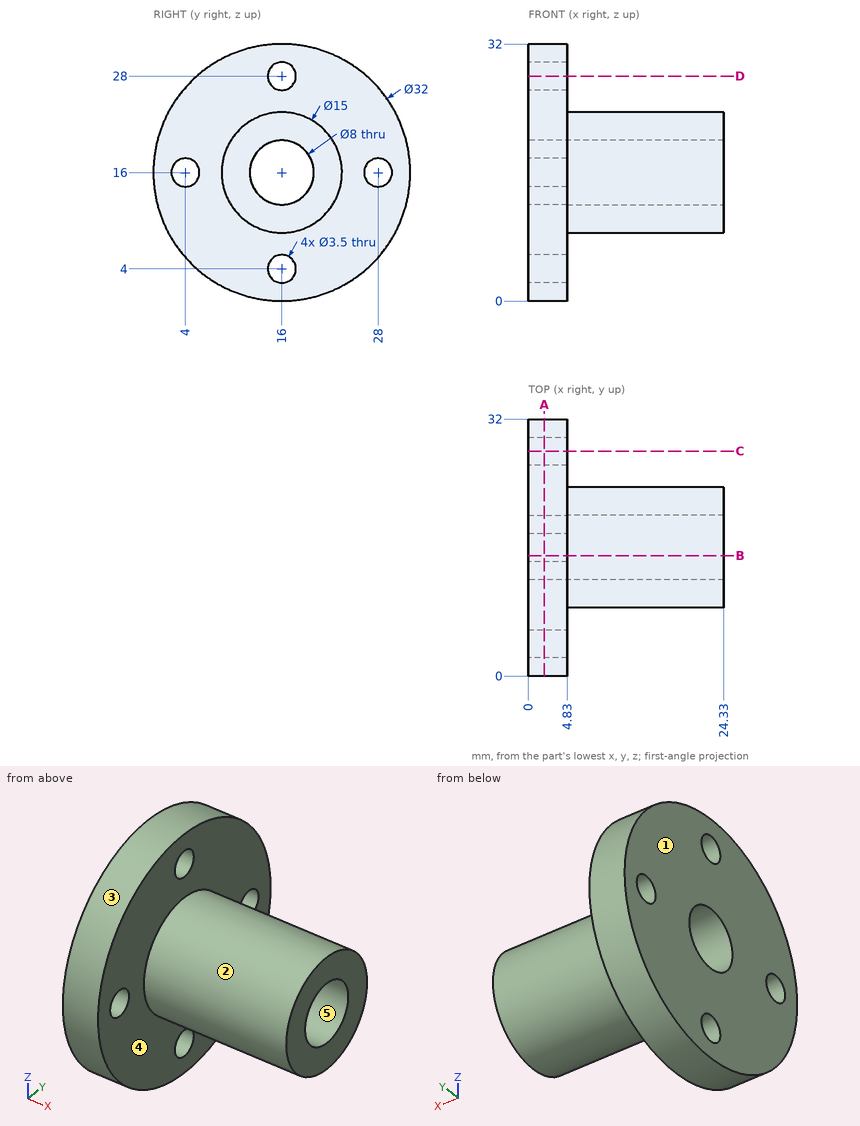
Could you check a few things on this drawing? It's one solid part, dimensions in mm from its lowest x, y, z. A direction names the side the tool comes from. Round coordinates to 2 decimals unless told otherwise and drop trailing zeros. Write each loop counter-clockwise with the first axis right and the second up, starting at its lowest first coordinate (ties: lowest second). Pieces come first, ordered by that corner, then holes. Notation, with made-up numbers: M 16,16.25 L 68,16.25 A23 ccw 68,44.25 Z; hole C -28,60.25 d11. An arc over 180 degrees is marked long. Answer as CSV lines item,"result". Start each with the question number.
1. Suppose I cut it at A-A on x = 2. Write out the boundary of the cut face in (y, z).
2. Suppose I cut it at C-C on y = 28. Write out the boundary of the cut face in (x, z).
3. I'm going to push flat-ended pins straight in: pin 1 Ø5 at (x, z) = (17, 20) entering from +Y; pin 2 Ø12 at (x, y) = (15, 7) entering from +Z; pin 3 Ø4 at (y, z) = (4, 16) entering from +X. Where does each tip first touch, or does it pass through?
4. Suppose I cut it at B-B on y = 15. Write out the boundary of the cut face in (x, z).
5. On a 3-axis mill with a long thin cutter (end or side, diameter ignored), from which of +Z, -Z, +X, -X, +Y, -Y can I reach the whole of each face in a straight line? I mean the marked faces 1 and 2. Say none if no direction works.
6. I need wall thicknesses on probe 1 along Z at (x, y) = (3.05, 16); probe 2 along X at (y, z) = (21.5, 7); probe 3 along Y at (x, z) = (2.25, 27). Which ranges of each line are inside material? Lowest first, please.
7. Thinking about a two-plate mould opening in Z: for the marked faces 3, 4 and 5, which applies, released by +Z, released by -Z, zero draft, split by the parting line, or undercut?
Check result:
1,outline,"C 16,16 d32; hole C 4,16 d3.5; hole C 16,16 d8; hole C 16,4 d3.5; hole C 16,28 d3.5; hole C 28,16 d3.5"
2,outline,"M 0,5.42 L 4.83,5.42 L 4.83,14.25 L 0,14.25 Z; M 0,17.75 L 4.83,17.75 L 4.83,26.58 L 0,26.58 Z"
3,pin 1,"stops at y = 23.35"
3,pin 2,"stops at z = 22.87"
3,pin 3,"stops at x = 4.83"
4,outline,"M 0,0.03 L 4.83,0.03 L 4.83,2.56 L 0,2.56 Z; M 0,5.44 L 4.83,5.44 L 4.83,8.57 L 24.33,8.57 L 24.33,12.13 L 0,12.13 Z; M 0,19.87 L 24.33,19.87 L 24.33,23.43 L 4.83,23.43 L 4.83,26.56 L 0,26.56 Z; M 0,29.44 L 4.83,29.44 L 4.83,31.97 L 0,31.97 Z"
5,face 1,"+Z, -Z, -X, +Y, -Y"
5,face 2,"+X"
6,probe 1,"z = 0 to 2.25, 5.75 to 12, 20 to 26.25, 29.75 to 32"
6,probe 2,"x = 0 to 4.83"
6,probe 3,"y = 4.38 to 14.56, 17.44 to 27.62"
7,face 3,"split by the parting line"
7,face 4,"zero draft"
7,face 5,"undercut"
